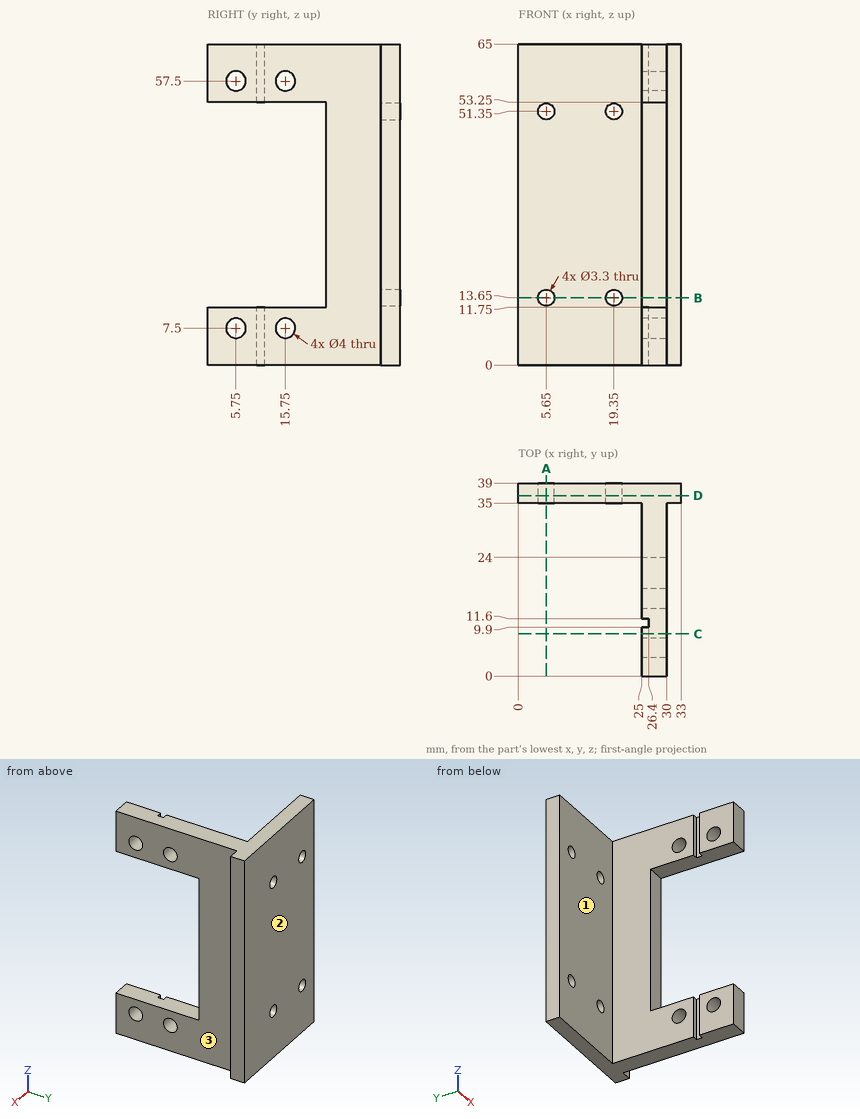
Answer from the drawing. Dimensions are ordinates in mm from the lowest x, y and z of the part. A direction names the side the tool comes from. Coordinates: 2 decimals unless noted, no trailing zeros. Order: outer loops, then holes, each group sorted by start corner. A loop starts at its lowest first (then second) coordinate and runs counter-clockwise, first axis right, second up. Notation, with made-up numbers: (14.5, 41.5) - (29.5, 41.5) arc R21 cw to (29.5, 64.5) - close; hole circle Ø3 at (77.25, 78). An arc over 180 degrees is marked (long way). Answer as a JSON object with one key per item and string values. Group by question number.
Item 1: Section C-C (y = 8.5) is taken. Give the vertices of the cut face in (x, z).
Item 2: A tool of negligible diameter and unlimited length cuts with its end or side. For the marked faces 1, 2 and 3, from which of +Z, -Z, +X, -X, +Y, -Y can it reach the whole face along a straight path? Write none if from no direction.
Item 3: Section A-A (x = 5.65) is taken. Give the vertices of the cut face in (y, z), plus the area to 3 significant figures.
Item 4: Section B-B (z = 13.65) is taken. Give the vertices of the cut face in (x, y), plus the area to 3 significant figures.
Item 5: Flat-ended cylindrical pins translate along their axes: P1, Ø8, axis at y = 3.5, z = 60, coming from the -X side; P2, Ø2, axis at x = 5.65, z = 51.35, coming from the +Y side; P3, Ø0.5, axis at y = 11, z = 3.5, coming from the -X side; P4, Ø4, axis at x = 5.65, z = 13.65, coming from the -Y side. Find the tip coordinate at first contact, or state that the pin passes through.
Item 6: Consider probe 1 along X at (y, z) = (37.7, 13.65); probe 2 along Y at (x, z) = (27.2, 7.5); probe 3 along X at (y, z) = (11.5, 8). Determine where each line is inside the solid, lowest interval first. Write a range as from..to.
Item 7: Section D-D (y = 36.5) is taken. Give the vertices of the cut face in (x, z).
Results are:
{
 "1": {"outline": "(25, 0) - (30, 0) - (30, 11.75) - (25, 11.75) - close; (25, 53.25) - (30, 53.25) - (30, 65) - (25, 65) - close"},
 "2": {"face 1": "+Z, -Z, -X, -Y", "face 2": "+Z, -Z, +X, -X, +Y", "face 3": "+Z, -Z, +X, -Y"},
 "3": {"outline": "(35, 0) - (39, 0) - (39, 12) - (35, 12) - close; (35, 15.3) - (39, 15.3) - (39, 49.7) - (35, 49.7) - close; (35, 53) - (39, 53) - (39, 65) - (35, 65) - close", "area": "234 mm^2"},
 "4": {"outline": "(0, 35) - (4, 35) - (4, 39) - (0, 39) - close; (7.3, 35) - (17.7, 35) - (17.7, 39) - (7.3, 39) - close; (21, 35) - (25, 35) - (25, 24) - (30, 24) - (30, 35) - (33, 35) - (33, 39) - (21, 39) - close", "area": "161 mm^2"},
 "5": {"P1": "stops at x = 25", "P2": "passes through", "P3": "stops at x = 26.4", "P4": "stops at y = 35"},
 "6": {"probe 1": "x = 0..4, 7.3..17.7, 21..33", "probe 2": "y = 0..3.75, 7.75..13.75, 17.75..39", "probe 3": "x = 26.4..30"},
 "7": {"outline": "(0, 0) - (33, 0) - (33, 65) - (0, 65) - close; hole circle Ø3.3 at (5.65, 13.65); hole circle Ø3.3 at (5.65, 51.35); hole circle Ø3.3 at (19.35, 13.65); hole circle Ø3.3 at (19.35, 51.35)"}
}
